For this review, take the finished solid that the model builds, in its own axes (mm). A direction names the side the tool comes from. Coordinates: 2 decimals unless noted, no trailing zeros. Write each loop counter-clockwise with the first axis right and the second up, starting at its lowest first coordinate (ties: lowest second). Pieces come first, ordered by that corner, then holes. Notation, with made-up numbers: (43, -13) - (102, -13) arc R33 cw to (102, 20) - close; hole circle Ø8 at (48, -17). An arc over 180 degrees is marked (long way). Write each question's results on one line, items separated by ' | '.
from build123d import *

# Parameters (mm, degrees)
SKETCH1_R           = 2
BOSS_EXTRUDE1_DEPTH = 6.7
CHAMFER1_SIZE       = 0.5
BOSS_EXTRUDE2_DEPTH = 2
CHAMFER2_SIZE       = 0.2


with BuildPart() as part:
    # Sketch1 → Boss-Extrude1 (new body)
    with BuildSketch(Plane.XY):
        Circle(SKETCH1_R)
    extrude(amount=BOSS_EXTRUDE1_DEPTH)

    # Chamfer1
    chamfer1_edges = [part.edges().sort_by_distance(p)[0] for p in [
        (-2, 0, 6.7),
    ]]
    chamfer(chamfer1_edges, length=CHAMFER1_SIZE)

    # Sketch2 → Boss-Extrude2 (add)
    with BuildSketch(Plane(origin=(0, 0, 0), x_dir=(-1, 0, 0), z_dir=(0, 0, -1))):
        Polygon((0.124813216, -2.884051836), (2.560068764, -1.333934502), (2.435255548, 1.550117334), (-0.124813216, 2.884051836), (-2.560068764, 1.333934502), (-2.435255548, -1.550117334), align=None)
    extrude(amount=BOSS_EXTRUDE2_DEPTH)

    # Chamfer2
    chamfer2_edges = [part.edges().sort_by_distance(p)[0] for p in [
        (1.155221166, -2.217084585, -2),
        (-1.34244099, -2.108993169, -2),
        (-2.497662156, 0.108091416, -2),
        (-1.155221166, 2.217084585, -2),
        (1.34244099, 2.108993169, -2),
        (2.497662156, -0.108091416, -2),
    ]]
    chamfer(chamfer2_edges, length=CHAMFER2_SIZE)


solid = part.part
Q1. Take a section at B-B on z = -1. State the section outline as (x, y) points, plus the area to 3 significant figures.
Results found:
outline: (-2.56, -1.33) - (-0.12, -2.88) - (2.44, -1.55) - (2.56, 1.33) - (0.12, 2.88) - (-2.44, 1.55) - close | area: 21.7 mm2
Q2. For faces 1 (the face through (2, -1, 0)), 2 (the face through (0, 0, -2)), list the 3-axis set-ups (+Z, -Z, +X, -X, +Y, -Y) from which the entire face can be reached by the end or side of a thin tool; tool diameter is ignored.
Results found:
face 1: +Z | face 2: -Z, +X, -X, +Y, -Y
Q3. Take a section at C-C on y = 0. State the section outline as (x, z) points, plus the area to 3 significant figures.
Results found:
outline: (-2.5, -1.8) - (-2.3, -2) - (2.3, -2) - (2.5, -1.8) - (2.5, 0) - (2, 0) - (2, 6.2) - (1.5, 6.7) - (-1.5, 6.7) - (-2, 6.2) - (-2, 0) - (-2.5, 0) - close | area: 36.5 mm2
Q4. Take a section at A-A on x = 0. State the section outline as (y, z) points.
Results found:
outline: (-2.82, -1.8) - (-2.59, -2) - (2.59, -2) - (2.82, -1.8) - (2.82, 0) - (2, 0) - (2, 6.2) - (1.5, 6.7) - (-1.5, 6.7) - (-2, 6.2) - (-2, 0) - (-2.82, 0) - close
Q5. Take a section at D-D on z = 6. State the section outline as (x, y) points, plus the area to 3 significant figures.
Results found:
outline: circle Ø4 at (0, 0) | area: 12.6 mm2
Q6. For pin 1 (1 mm diameter, centred on y = 0.5, z = 5, fed in from -X); pin 2 (1 mm diameter, centred on x = 0, z = 1, fed in from -Y), all flat-tipped, find the tip position at first contact; note any pin that passes through.
Results found:
pin 1: x = -2 | pin 2: y = -2
Q7. Wall thickness on line 1 along X through (y, z) = (0.1, 4.25); line 2 along Z through (x, y) = (2.2, 0.95); line 3 along Y through (x, z) = (-0.45, 5.25): over which ranges is each line inside the solid? List them lowest first. Write a range as from..to.
Results found:
line 1: -2..2 | line 2: -2..0 | line 3: -1.95..1.95
